Source: CAD feature listing. Evaluate the final solid. Frame: model axes, mm. A direction names the side the tool comes from. Give positions to 0.01 mm unless a question says otherwise; leave off trailing zeros. Order: outer loops, then holes, each group sorted by start corner. A loop starts at its lowest first (then second) coordinate and runs counter-clockwise, first axis right, second up.
from build123d import *

# Parameters (mm, degrees)
F1_DEPTH = 4
F2_W     = 3
F2_H     = 105
F2_W_2   = 70
F2_H_2   = 3
F2_R     = 1.9
F3_DEPTH = 5
F4_R     = 1.5
F5_DEPTH = 25
F6_DEPTH = 25
F7_DEPTH = 25
F8_DEPTH = 25


with BuildPart() as f1:
    # F0 (on Top) → F1 (new body)
    with BuildSketch(Plane.XY):
        with BuildLine():
            Line((41, 62.5), (-41, 62.5))
            ThreePointArc((-41, 62.5), (-43.8284271247, 61.3284271247), (-45, 58.5))
            Line((-45, 58.5), (-45, -58.5))
            ThreePointArc((-45, -58.5), (-43.8284271247, -61.3284271247), (-41, -62.5))
            Line((-41, -62.5), (41, -62.5))
            ThreePointArc((41, -62.5), (43.8284271247, -61.3284271247), (45, -58.5))
            Line((45, -58.5), (45, 58.5))
            ThreePointArc((45, 58.5), (43.8284271247, 61.3284271247), (41, 62.5))
        make_face()
    extrude(amount=F1_DEPTH)

    # F2 (on face) → F3 (join)
    with BuildSketch(Plane.XY.offset(4)):
        with Locations((43.5, 0)):
            Rectangle(F2_W, F2_H)
        with Locations((0, -61)):
            Rectangle(F2_W_2, F2_H_2)
        with Locations((-43.5, 0)):
            Rectangle(F2_W, F2_H)
        with Locations((0, 61)):
            Rectangle(F2_W_2, F2_H_2)
        with BuildLine():
            Line((-45, 58.5), (-45, 52.5))
            Line((-45, 52.5), (-42, 52.5))
            Line((-42, 52.5), (-38, 52.5))
            ThreePointArc((-38, 52.5), (-35.8786796564, 53.3786796564), (-35, 55.5))
            Line((-35, 55.5), (-35, 59.5))
            Line((-35, 59.5), (-35, 62.5))
            Line((-35, 62.5), (-41, 62.5))
            ThreePointArc((-41, 62.5), (-43.8284271247, 61.3284271247), (-45, 58.5))
        make_face()
        with Locations((-40, 57.5)):
            Circle(F2_R, mode=Mode.SUBTRACT)
        with BuildLine():
            Line((41, 62.5), (35, 62.5))
            Line((35, 62.5), (35, 59.5))
            Line((35, 59.5), (35, 55.5))
            ThreePointArc((35, 55.5), (35.8786796564, 53.3786796564), (38, 52.5))
            Line((38, 52.5), (42, 52.5))
            Line((42, 52.5), (45, 52.5))
            Line((45, 52.5), (45, 58.5))
            ThreePointArc((45, 58.5), (43.8284271247, 61.3284271247), (41, 62.5))
        make_face()
        with Locations((40, 57.5)):
            Circle(F2_R, mode=Mode.SUBTRACT)
        with BuildLine():
            Line((35, -59.5), (35, -62.5))
            Line((35, -62.5), (41, -62.5))
            ThreePointArc((41, -62.5), (43.8284271247, -61.3284271247), (45, -58.5))
            Line((45, -58.5), (45, -52.5))
            Line((45, -52.5), (42, -52.5))
            Line((42, -52.5), (38, -52.5))
            ThreePointArc((38, -52.5), (35.8786796564, -53.3786796564), (35, -55.5))
            Line((35, -55.5), (35, -59.5))
        make_face()
        with Locations((40, -57.5)):
            Circle(F2_R, mode=Mode.SUBTRACT)
        with BuildLine():
            Line((-42, -52.5), (-45, -52.5))
            Line((-45, -52.5), (-45, -58.5))
            ThreePointArc((-45, -58.5), (-43.8284271247, -61.3284271247), (-41, -62.5))
            Line((-41, -62.5), (-35, -62.5))
            Line((-35, -62.5), (-35, -59.5))
            Line((-35, -59.5), (-35, -55.5))
            ThreePointArc((-35, -55.5), (-35.8786796564, -53.3786796564), (-38, -52.5))
            Line((-38, -52.5), (-42, -52.5))
        make_face()
        with Locations((-40, -57.5)):
            Circle(F2_R, mode=Mode.SUBTRACT)
    extrude(amount=F3_DEPTH)

    # F4
    f4_edges = [f1.edges().sort_by_distance(p)[0] for p in [
        (0, 62.5, 0),
        (-43.828427, 61.328427, 0),
        (-45, 0, 0),
        (-43.828427, -61.328427, 0),
        (0, -62.5, 0),
        (43.828427, -61.328427, 0),
        (45, 0, 0),
        (43.828427, 61.328427, 0),
    ]]
    fillet(f4_edges, radius=F4_R)

    # F5 (cut): a face of the model
    f5_faces = [f1.faces().sort_by_distance(p)[0] for p in [
        (-40, 57.5, 4),
    ]]
    extrude(f5_faces, amount=-F5_DEPTH, mode=Mode.SUBTRACT)

    # F6 (cut): a face of the model
    f6_faces = [f1.faces().sort_by_distance(p)[0] for p in [
        (40, 57.5, 4),
    ]]
    extrude(f6_faces, amount=-F6_DEPTH, mode=Mode.SUBTRACT)

    # F7 (cut): a face of the model
    f7_faces = [f1.faces().sort_by_distance(p)[0] for p in [
        (40, -57.5, 4),
    ]]
    extrude(f7_faces, amount=-F7_DEPTH, mode=Mode.SUBTRACT)

    # F8 (cut): a face of the model
    f8_faces = [f1.faces().sort_by_distance(p)[0] for p in [
        (-40, -57.5, 4),
    ]]
    extrude(f8_faces, amount=-F8_DEPTH, mode=Mode.SUBTRACT)


solid = f1.part
1) Section query A-A on z = 7.75. Output: boundary loops of the cut face in (x, y).
Checks:
outline: (-45, -58.5) arc R4 ccw to (-41, -62.5) - (41, -62.5) arc R4 ccw to (45, -58.5) - (45, 58.5) arc R4 ccw to (41, 62.5) - (-41, 62.5) arc R4 ccw to (-45, 58.5) - close; hole (-42, -52.5) - (-38, -52.5) arc R3 cw to (-35, -55.5) - (-35, -59.5) - (35, -59.5) - (35, -55.5) arc R3 cw to (38, -52.5) - (42, -52.5) - (42, 52.5) - (38, 52.5) arc R3 cw to (35, 55.5) - (35, 59.5) - (-35, 59.5) - (-35, 55.5) arc R3 cw to (-38, 52.5) - (-42, 52.5) - close; hole circle Ø3.8 at (-40, -57.5); hole circle Ø3.8 at (-40, 57.5); hole circle Ø3.8 at (40, -57.5); hole circle Ø3.8 at (40, 57.5)
2) Section query B-B on y = -43. Output: boundary loops of the cut face in (x, z).
Checks:
outline: (-45, 1.5) arc R1.5 ccw to (-43.5, 0) - (43.5, 0) arc R1.5 ccw to (45, 1.5) - (45, 9) - (42, 9) - (42, 4) - (-42, 4) - (-42, 9) - (-45, 9) - close
3) Reachability of faces 1 (the face through (-35, 57, 6)), 2 (the face through (1, 62.5, 5)) from +Z, -Z, +X, -X, +Y, -Y: full face, straight path, thin tool, end or side. Return the list, or none.
Checks:
face 1: +Z
face 2: +Z, -Z, +X, -X, +Y
4) Pull-direction query (X, two-part tool) for faces 3 (the face through (-43.859, -61.297, 5.198)), 4 (the face through (0, 59.5, 6)), 5 (the face through (-1, 1, 0)); classes: +X half, -X half, draft (parallel to the pull), parting line (faces both ways), or undercut.
Checks:
face 3: -X half
face 4: undercut
face 5: draft
5) Section query C-C on x = -29.5. Output: boundary loops of the cut face in (y, z).
Checks:
outline: (-62.5, 1.5) arc R1.5 ccw to (-61, 0) - (61, 0) arc R1.5 ccw to (62.5, 1.5) - (62.5, 9) - (59.5, 9) - (59.5, 4) - (-59.5, 4) - (-59.5, 9) - (-62.5, 9) - close
6) Ray query, L1, parallel to Y at x = -40, z = 1.3; L2, parallel to Y at x = -40, z = 5.8; L3, parallel to X at y = 25, z = 8.75. Return the intervals inside material, ascending.
Checks:
L1: y = -62.49 to -59.4, -55.6 to 55.6, 59.4 to 62.49
L2: y = -62.5 to -59.4, -55.6 to -52.5, 52.5 to 55.6, 59.4 to 62.5
L3: x = -45 to -42, 42 to 45
7) First-contact query: pin 1 Ø6 at (x, y) = (-14, 9.5) entering from -Z; pin 2 Ø4 at (x, y) = (21.5, 28) entering from +Z. Flat tips, straight axial feed; report the tip coordinate or a pass-through.
Checks:
pin 1: stops at z = 0
pin 2: stops at z = 4
